Can you work these out from the model? Positions are in its coordinate system, mm. A direction names the side the tool comes from. Give positions to 0.01 mm unless a question says otherwise; leave off trailing zeros. Loops run counter-clockwise (first coordinate to the right, second up) from the corner with the lowest first, then second, coordinate; pieces in that order, holes last. Notation, with made-up numbers: (39.5, 76.5) - (86.5, 76.5) arc R26 ccw to (86.5, 115.5) - close; hole circle Ø4 at (-35.75, -32.5). An arc over 180 degrees is marked (long way). Answer in a Markdown table with one row per item.
from build123d import *

# Parameters (mm, degrees)
BOSS_EXTRUDE1_DEPTH     = 914.4
SHELL1_T                = -19.05
BOSS_EXTRUDE2_REACH     = 1484.708
SKETCH2_W               = 876.3
SKETCH2_H               = 234.95
SHELL2_START            = 19.05
SHELL2_DEPTH            = 876.3
SKETCH6_W               = 50.8
SKETCH6_H               = 50.8
SKETCH6_W_2             = 25.4
SKETCH6_H_2             = 25.4
BOSS_EXTRUDE3_DEPTH     = 457.2
SKETCH7_W               = 50.8
SKETCH7_H               = 50.8
BOSS_EXTRUDE4_DEPTH     = 609.6
CUT_EXTRUDE2_DEPTH      = 1483.708003115
CUT_EXTRUDE2_DEPTH_BACK = 1483.708003115
SKETCH9_W               = 696
SKETCH9_H               = 388


# Read off the part's stored shape, not the designer's step: Shell2
with BuildPart() as part:
    # Sketch1 → Boss-Extrude1 (new body)
    with BuildSketch(Plane.XY):
        Polygon((0, 0), (711.2, 0), (545.48790353, 939.8), (0, 939.8), align=None)
    extrude(amount=BOSS_EXTRUDE1_DEPTH)

    # Shell1
    shell1_openings = [part.faces().sort_by_distance(p)[0] for p in [
        (628.343951765, 469.9, 457.2),
    ]]
    offset(amount=SHELL1_T, openings=shell1_openings, kind=Kind.INTERSECTION)

    # Boss-Extrude2: up to this plane
    boss_extrude2_end = Plane(origin=(711.2, 0, 914.4), z_dir=(-0.9848077530122075, -0.1736481776669338, 0))
    # Sketch2 → Boss-Extrude2 (add, up to the surface)
    with BuildSketch(Plane(origin=(19.05, 0, 0), x_dir=(0, 0, -1), z_dir=(1, 0, 0)), mode=Mode.PRIVATE) as boss_extrude2_sk1:
        with Locations((-457.2, 803.275)):
            Rectangle(SKETCH2_W, SKETCH2_H)
    boss_extrude2_tool1 = split(extrude(boss_extrude2_sk1.sketch, amount=BOSS_EXTRUDE2_REACH, mode=Mode.PRIVATE), bisect_by=boss_extrude2_end, keep=Keep.BOTH, mode=Mode.PRIVATE)
    add(boss_extrude2_tool1.solids().sort_by_distance((19.05, 803.275, 457.2))[0])

    # Shell2 outline → Shell2 (cut)
    with BuildSketch(Plane.XY.offset(SHELL2_START)):
        Polygon((19.05, 920.75), (19.05, 685.8), (570.931079674, 685.8), (529.503055556, 920.75), align=None)
    extrude(amount=SHELL2_DEPTH, mode=Mode.SUBTRACT)

    # Sketch6 → Boss-Extrude3 (add)
    # profile 1 of 4: a face of its own
    with BuildSketch(Plane.XZ):
        with Locations((685.8, 889)):
            Rectangle(SKETCH6_W, SKETCH6_H)
        with Locations((685.8, 889)):
            Rectangle(SKETCH6_W_2, SKETCH6_H_2, mode=Mode.SUBTRACT)
    # profile 2 of 4: a face of its own
    with BuildSketch(Plane.XZ):
        with Locations((685.8, 25.4)):
            Rectangle(SKETCH6_W, SKETCH6_H)
        with Locations((685.8, 25.4)):
            Rectangle(SKETCH6_W_2, SKETCH6_H_2, mode=Mode.SUBTRACT)
    # profile 3 of 4: a face of its own
    with BuildSketch(Plane.XZ):
        with Locations((25.4, 25.4)):
            Rectangle(SKETCH6_W, SKETCH6_H)
        with Locations((25.4, 25.4)):
            Rectangle(SKETCH6_W_2, SKETCH6_H_2, mode=Mode.SUBTRACT)
    # profile 4 of 4: a face of its own
    with BuildSketch(Plane.XZ):
        with Locations((25.4, 889)):
            Rectangle(SKETCH6_W, SKETCH6_H)
        with Locations((25.4, 889)):
            Rectangle(SKETCH6_W_2, SKETCH6_H_2, mode=Mode.SUBTRACT)
    extrude(amount=BOSS_EXTRUDE3_DEPTH)

    # Sketch7 → Boss-Extrude4 (add)
    with BuildSketch(Plane(origin=(50.8, 0, 0), x_dir=(0, 0, -1), z_dir=(1, 0, 0))):
        with Locations((-889, -431.8)):
            Rectangle(SKETCH7_W, SKETCH7_H)
        with Locations((-25.4, -431.8)):
            Rectangle(SKETCH7_W, SKETCH7_H)
        with Locations((-889, -88.9)):
            Rectangle(SKETCH7_W, SKETCH7_H)
        with Locations((-25.4, -88.9)):
            Rectangle(SKETCH7_W, SKETCH7_H)
    extrude(amount=BOSS_EXTRUDE4_DEPTH)

    # Sketch9 → Cut-Extrude2 (cut, two sides: drawn at the far end of the back side and taken through both)
    with BuildSketch(Plane(origin=(19.05, 0, 0), x_dir=(0, 0, -1), z_dir=(1, 0, 0)).offset(-CUT_EXTRUDE2_DEPTH_BACK)):
        with Locations((-457.4, 388.05)):
            Rectangle(SKETCH9_W, SKETCH9_H)
    extrude(amount=CUT_EXTRUDE2_DEPTH + CUT_EXTRUDE2_DEPTH_BACK, mode=Mode.SUBTRACT)


solid = part.part
Q1. If we mould it in two halves opening along X, with no side actions, what happens to faces 5 (the face through (19.05, 677, 451)), 6 (the face through (351, -73, 50.8)), 7 (the face through (572.72, 785.36, 527.07))? For each: released by +X, released by -X, zero draft, split by the parting line, or undercut.
Checked values:
| item | result |
|---|---|
| face 5 | undercut |
| face 6 | zero draft |
| face 7 | released by +X |
Q2. On a 3-axis mill with a long thin cutter (end or side, diameter ignored), from which of +Z, -Z, +X, -X, +Y, -Y can I reach the whole of each face in a straight line? I mean faces 1 (the face through (550.507, 801.63, 451.066)), 2 (the face through (351, -79, 863.6)), 3 (the face through (359, 19.05, 451)), 4 (the face through (50.8, -258, 25)). Say none if no direction works.
Checked values:
| item | result |
|---|---|
| face 1 | none |
| face 2 | +X, -X, -Y |
| face 3 | +X |
| face 4 | +Z, -Z |
Q3. Imagine slicing it at D-D, the plane y = 529. Write out the boundary of the cut face in (x, z).
Checked values:
| item | result |
|---|---|
| outline | (0, 0) - (617.92, 0) - (617.92, 19.05) - (19.05, 19.05) - (19.05, 109.4) - (0, 109.4) - close; (0, 805.4) - (19.05, 805.4) - (19.05, 895.35) - (617.92, 895.35) - (617.92, 914.4) - (0, 914.4) - close |
Q4. Imagine slicing it at B-B, the plane y = -149. Count the separate pieces of the cut face and the enclosed holes in it, and give its area (3 significant figures).
Checked values:
| item | result |
|---|---|
| separate pieces | 4 |
| enclosed holes | 4 |
| area | 7,740 mm² |
Q5. If I drill on line 1 (Z direction, x = 314, y = 778.5); line 2 (Y direction, x = 337.5, z = 704.5); line 3 (X direction, y = 157.5, z = 96.5), over which ranges is the centre line in solid material (lowest first)? Write a range as [from, to].
Checked values:
| item | result |
|---|---|
| line 1 | z = [0, 19.05], [895.35, 914.4] |
| line 2 | y = [0, 19.05], [920.75, 939.8] |
| line 3 | x = [0, 19.05] |
Q6. For pin 1 (1.5 mm diameter, centred on x = 503, z = 200, fed in from -Y); pin 2 (6 mm diameter, centred on y = 65.5, z = 212, fed in from +X), each with a flat end and sliding along its axis, tell me the tip position at first contact or that it passes through.
Checked values:
| item | result |
|---|---|
| pin 1 | stops at y = 0 |
| pin 2 | stops at x = 19.05 |
Q7. Imagine slicing it at C-C, the plane z = 342.5. Write out the boundary of the cut face in (x, y), and give its area (3 significant figures).
Checked values:
| item | result |
|---|---|
| outline | (0, 0) - (711.2, 0) - (707.84, 19.05) - (19.05, 19.05) - (19.05, 194.05) - (0, 194.05) - close; (0, 582.05) - (19.05, 582.05) - (19.05, 920.75) - (529.5, 920.75) - (570.93, 685.8) - (590.27, 685.8) - (545.49, 939.8) - (0, 939.8) - close |
| area | 38,300 mm² |
Q8. Imagine slicing it at A-A, the plane x = 116.5. Write out the boundary of the cut face in (y, z).
Checked values:
| item | result |
|---|---|
| outline | (-457.2, 0) - (-406.4, 0) - (-406.4, 50.8) - (-457.2, 50.8) - close; (-457.2, 863.6) - (-406.4, 863.6) - (-406.4, 914.4) - (-457.2, 914.4) - close; (-114.3, 0) - (-63.5, 0) - (-63.5, 50.8) - (-114.3, 50.8) - close; (-114.3, 863.6) - (-63.5, 863.6) - (-63.5, 914.4) - (-114.3, 914.4) - close; (0, 0) - (939.8, 0) - (939.8, 914.4) - (0, 914.4) - close; hole (19.05, 19.05) - (920.75, 19.05) - (920.75, 895.35) - (19.05, 895.35) - close |
